Can you work these out from the drawing? Everything is in mm from the part's minimum corner. A direction names the side the tool comes from. Give positions to 0.01 mm unless a question says otherwise; leave off trailing zeros. Loops run counter-clockwise (first coordinate to the right, second up) from the corner with the lowest first, then second, coordinate; pieces in that order, holes last.
Q1. If we section it at C-C (z = 27): Please give me the cut outline in (x, y), plus the area to 3 significant figures.
Q2. If we section it at B-B (y = 12): Please give me the cut outline in (x, z), plus the area to 3 significant figures.
Q3. If we section it at D-D (y = 34): Please give me the cut outline in (x, z).
Q4. We'd pull the mould along X, two halves only. Please class the marked faces 1, 2 and 3: +X half, -X half, draft (parallel to the pull), parting line (faces both ways), or undercut.
Q5. I need wall thicknesses on line 1 (X direction, y = 1, z = 27); line 2 (Z direction, x = 12.5, y = 1.6); line 3 (Z direction, x = 12, y = 2). Which ranges of each line are inside material? Lowest first, please.
Q6. For the marked faces 4, 5, 6 and 7, which set-ups out of +Z, -Z, +X, -X, +Y, -Y let a thin tool reach every point of the face, with its end or its side?
Q7. If we section it at A-A (x = 12.5): Please give me the cut outline in (y, z).
Q8. Will these pins go through, and if not, where does the flat tip stop? P1, Ø2, axis at y = 29, z = 18.5, coming from the +X side; P2, Ø5, axis at x = 12.5, z = 9, coming from the +Y side; P3, Ø16, axis at x = 85, z = 13, coming from the +Y side.
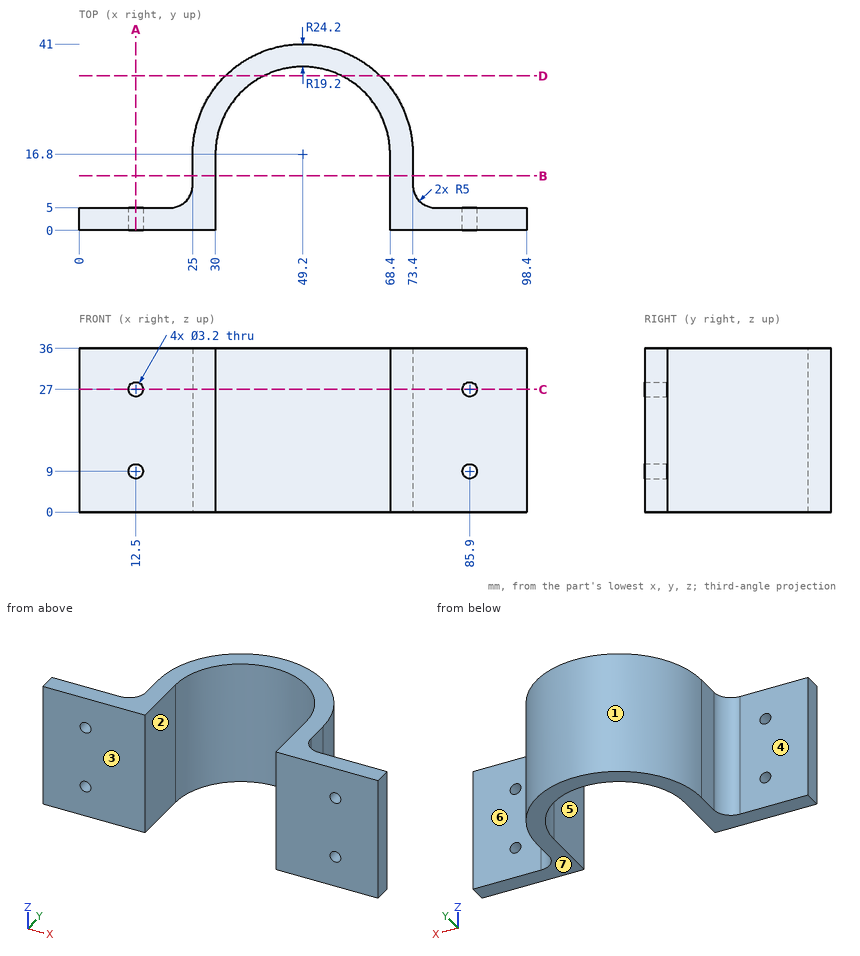
Check sheet entries:
1. outline: (0, 0) - (10.9, 0) - (10.9, 5) - (0, 5) - close; (14.1, 0) - (30, 0) - (30, 16.8) arc R19.2 cw to (68.4, 16.8) - (68.4, 0) - (84.3, 0) - (84.3, 5) - (78.4, 5) arc R5 cw to (73.4, 10) - (73.4, 16.8) arc R24.2 ccw to (25, 16.8) - (25, 10) arc R5 cw to (20, 5) - (14.1, 5) - close; (87.5, 0) - (98.4, 0) - (98.4, 5) - (87.5, 5) - close
1. area: 738 mm2
2. outline: (25, 0) - (30, 0) - (30, 36) - (25, 36) - close; (68.4, 0) - (73.4, 0) - (73.4, 36) - (68.4, 36) - close
2. area: 360 mm2
3. outline: (32.18, 0) - (40.67, 0) - (40.67, 36) - (32.18, 36) - close; (57.73, 0) - (66.22, 0) - (66.22, 36) - (57.73, 36) - close
4. face 1: parting line
4. face 2: undercut
4. face 3: draft
5. line 1: x = 0 to 10.9, 14.1 to 30, 68.4 to 84.3, 87.5 to 98.4
5. line 2: z = 0 to 7.4, 10.6 to 25.4, 28.6 to 36
5. line 3: z = 0 to 7.48, 10.52 to 25.48, 28.52 to 36
6. face 4: +Z, -Z, -X, +Y
6. face 5: +Z, -Z, -Y
6. face 6: +Z, -Z, +X, +Y
6. face 7: -Z, +X, -X, +Y, -Y
7. outline: (0, 0) - (5, 0) - (5, 7.4) - (0, 7.4) - close; (0, 10.6) - (5, 10.6) - (5, 25.4) - (0, 25.4) - close; (0, 28.6) - (5, 28.6) - (5, 36) - (0, 36) - close
8. P1: stops at x = 70.65
8. P2: stops at y = 5
8. P3: stops at y = 5.2
